The model under review builds one solid part; all positions refer to its coordinate system, in mm. A direction names the side the tool comes from. Round coordinates to 2 decimals unless told otherwise and drop trailing zeros. Order: outer loops, then holes, each group sorted by start corner. A loop starts at its lowest first (then second) coordinate and runs counter-clockwise, first axis right, second up. Notation, with made-up numbers: (82, 77) -> (93, 77) arc R14 ccw to (93, 95) -> close; hole circle Ø5 at (17.25, 57). An arc over 180 degrees is marked (long way). Use a Markdown table: item, result. Add a question column.
```python
from build123d import *

# Parameters (mm, degrees)
SKETCH1_R                      = 30
BOSS_EXTRUDE1_DEPTH            = 31.16
CUT_EXTRUDE1_DEPTH             = 29.16
CBORE_FOR_M4_SHCS1_D           = 4.5
CBORE_FOR_M4_SHCS1_CBORE_D     = 8
CBORE_FOR_M4_SHCS1_CBORE_DEPTH = 11
SKETCH7_R                      = 2.3495
CUT_EXTRUDE2_DEPTH             = 29.16
SKETCH9_R                      = 2.6162
CUT_EXTRUDE3_DEPTH             = 6.35


with BuildPart() as part:
    # Sketch1 → Boss-Extrude1 (new body)
    with BuildSketch(Plane(origin=(0, 0, 0), x_dir=(1, 0, 0), z_dir=(0, 1, 0))):
        with Locations(Location((0, 0, 0), (0, 0, 270))):
            Circle(SKETCH1_R)
    extrude(amount=BOSS_EXTRUDE1_DEPTH)

    # Sketch2 → Cut-Extrude1 (cut)
    with BuildSketch(Plane(origin=(0, 31.16, 0), x_dir=(1, 0, 0), z_dir=(0, 1, 0))):
        with BuildLine():
            Line((-6.184658438, -2), (-13.75, -2))
            Line((-13.75, -2), (-13.75, 2))
            Line((-13.75, 2), (-6.184658438, 2))
            ThreePointArc((-6.184658438, 2), (0, 6.5), (6.184658438, 2))
            Line((6.184658438, 2), (13.75, 2))
            Line((13.75, 2), (13.75, -2))
            Line((13.75, -2), (6.184658438, -2))
            ThreePointArc((6.184658438, -2), (0, -6.5), (-6.184658438, -2))
        make_face()
    extrude(amount=-CUT_EXTRUDE1_DEPTH, mode=Mode.SUBTRACT)

    # CBORE for M4 SHCS1 (through all)
    with Locations(Plane(origin=(0, 31.16, 0), x_dir=(1, 0, 0), z_dir=(0, 1, 0))):
        with Locations((0, 19), (-16.454482672, 9.5), (-16.454482672, -9.5), (0, -19), (16.454482672, -9.5), (16.454482672, 9.5)):
            CounterBoreHole(CBORE_FOR_M4_SHCS1_D / 2, CBORE_FOR_M4_SHCS1_CBORE_D / 2, CBORE_FOR_M4_SHCS1_CBORE_DEPTH)

    # Sketch7 → Cut-Extrude2 (cut)
    with BuildSketch(Plane(origin=(0, 31.16, 0), x_dir=(1, 0, 0), z_dir=(0, 1, 0))):
        with Locations(Location((-25.5, 0, 0), (0, 0, 270))):
            Circle(SKETCH7_R)
        with Locations(Location((-12.75, 22.083647797, 0), (0, 0, 270))):
            Circle(SKETCH7_R)
        with Locations(Location((12.75, 22.083647797, 0), (0, 0, 270))):
            Circle(SKETCH7_R)
        with Locations(Location((25.5, 0, 0), (0, 0, 270))):
            Circle(SKETCH7_R)
        with Locations(Location((12.75, -22.083647797, 0), (0, 0, 270))):
            Circle(SKETCH7_R)
        with Locations(Location((-12.75, -22.083647797, 0), (0, 0, 270))):
            Circle(SKETCH7_R)
    extrude(amount=-CUT_EXTRUDE2_DEPTH, mode=Mode.SUBTRACT)

    # Sketch9 → Cut-Extrude3 (cut)
    with BuildSketch(Plane(origin=(0, 31.16, 0), x_dir=(1, 0, 0), z_dir=(0, 1, 0))):
        with Locations(Location((-12.75, 22.083647797, 0), (0, 0, 270))):
            Circle(SKETCH9_R)
        with Locations(Location((12.75, 22.083647797, 0), (0, 0, 270))):
            Circle(SKETCH9_R)
        with Locations(Location((25.5, 0, 0), (0, 0, 270))):
            Circle(SKETCH9_R)
        with Locations(Location((12.75, -22.083647797, 0), (0, 0, 270))):
            Circle(SKETCH9_R)
        with Locations(Location((-12.75, -22.083647797, 0), (0, 0, 270))):
            Circle(SKETCH9_R)
        with Locations(Location((-25.5, 0, 0), (0, 0, 270))):
            Circle(SKETCH9_R)
    extrude(amount=-CUT_EXTRUDE3_DEPTH, mode=Mode.SUBTRACT)


solid = part.part
```
Q1. For faces 3 (the face through (18.113, 9.939, -11.021)), 4 (the face through (10, 17, -2)), list the 3-axis set-ups (+Z, -Z, +X, -X, +Y, -Y) from which the entire face can be reached by the end or side of a thin tool; tool diameter is ignored.
Q2. Add section C-C, the plane z = 0. Give the boundary of the cut face in (x, y).
Q3. For pin 1 (1 mm diameter, centred on y = 12, z = 10.5, fed in from -X); pin 2 (1.5 mm diameter, centred on x = -3, y = 10, fed in from +Z); pin 3 (3 mm diameter, centred on y = 16.5, z = 0.5, fed in from +X), all flat-tipped, find the tip position at first contact; note any pin that passes through.
Q4. Add section D-D, the plane z = -20.5. Give the boundary of the cut face in (x, y).
Q5. Add section B-B, the plane y = 13. Give the number of separate pieces and of enclosed holes in the cut face, then the cut area to 3 significant figures.
Q6. To check wall thickness, follow line 1 along X through (y, z) = (10.25, 0); line 2 along X through (y, z) = (22.5, -7.5); line 3 along X through (y, z) = (29, 0). State the ranges of each line that lie inside material, in increasing order.
Q7. Add section A-A, the plane x = 0. Give the boundary of the cut face in (y, z).
Q8. Draft analysis for pull direction Z (two halves, no side actions). For faces 1 (the face through (-6, 31.16, 6)), 2 (the face through (-12.63, 28.03, 19.47)), state which applies: released by +Z, released by -Z, zero draft, split by the parting line, or undercut.
Return value:
| question | item | result |
|---|---|---|
| 1 | face 3 | +Y, -Y |
| 1 | face 4 | +Y |
| 2 | outline | (-30, 0) -> (30, 0) -> (30, 31.16) -> (28.12, 31.16) -> (28.12, 24.81) -> (27.85, 24.81) -> (27.85, 2) -> (23.15, 2) -> (23.15, 24.81) -> (22.88, 24.81) -> (22.88, 31.16) -> (13.75, 31.16) -> (13.75, 2) -> (-13.75, 2) -> (-13.75, 31.16) -> (-22.88, 31.16) -> (-22.88, 24.81) -> (-23.15, 24.81) -> (-23.15, 2) -> (-27.85, 2) -> (-27.85, 24.81) -> (-28.12, 24.81) -> (-28.12, 31.16) -> (-30, 31.16) -> close |
| 3 | pin 1 | x = -28.28 |
| 3 | pin 2 | z = 29.92 |
| 3 | pin 3 | x = 30 |
| 4 | outline | (-21.9, 0) -> (-1.68, 0) -> (-1.68, 20.16) -> (-3.71, 20.16) -> (-3.71, 31.16) -> (-10.67, 31.16) -> (-10.67, 24.81) -> (-11.01, 24.81) -> (-11.01, 2) -> (-14.49, 2) -> (-14.49, 24.81) -> (-14.83, 24.81) -> (-14.83, 31.16) -> (-21.9, 31.16) -> close; (1.68, 0) -> (21.9, 0) -> (21.9, 31.16) -> (14.83, 31.16) -> (14.83, 24.81) -> (14.49, 24.81) -> (14.49, 2) -> (11.01, 2) -> (11.01, 24.81) -> (10.67, 24.81) -> (10.67, 31.16) -> (3.71, 31.16) -> (3.71, 20.16) -> (1.68, 20.16) -> close |
| 5 | separate pieces | 1 |
| 5 | enclosed holes | 13 |
| 5 | area | 2,440 mm² |
| 6 | line 1 | -30 to -27.85, -23.15 to -13.75, 13.75 to 23.15, 27.85 to 30 |
| 6 | line 2 | -29.05 to -19.92, -12.99 to 12.99, 19.92 to 29.05 |
| 6 | line 3 | -30 to -28.12, -22.88 to -13.75, 13.75 to 22.88, 28.12 to 30 |
| 7 | outline | (0, -30) -> (31.16, -30) -> (31.16, -23) -> (20.16, -23) -> (20.16, -21.25) -> (0, -21.25) -> close; (0, -16.75) -> (20.16, -16.75) -> (20.16, -15) -> (31.16, -15) -> (31.16, -6.5) -> (2, -6.5) -> (2, 6.5) -> (31.16, 6.5) -> (31.16, 15) -> (20.16, 15) -> (20.16, 16.75) -> (0, 16.75) -> close; (0, 21.25) -> (20.16, 21.25) -> (20.16, 23) -> (31.16, 23) -> (31.16, 30) -> (0, 30) -> close |
| 8 | face 1 | zero draft |
| 8 | face 2 | undercut |
